Build history of the part. All positions in model axes, mm. Face numbers are marked on the shaded views. A direction names the side the tool comes from. Give positions to 0.01 mm unless a question says otherwise; leave off trailing zeros. Order: outer loops, then holes, each group sorted by start corner. A loop starts at its lowest first (then second) coordinate and runs counter-clockwise, first axis right, second up. Notation, with made-up numbers: M -18,88.25 L 40,88.25 A24 cw 40,104.25 Z; hole C -7.75,81 d5. An arc over 180 degrees is marked long. Use CSV: the item, a comma, the result in double quotes. Start each with the question number.
Item 1: Which spindle directions (+Z, -Z, +X, -X, +Y, -Y) get a long thin tool onto all of the face, cutting with end or side? Do the marked faces 1 and 2. Say none if no direction does.
Item 2: Pin check, flat tips, straight feed: P1, Ø4, axis at x = -5, y = -9.5, coming from the -Z side; P2, Ø1.4, axis at y = 0, z = 2.5, coming from the -X side; P3, Ø1, axis at y = 25, z = 2.5, coming from the +X side. Stop position of each tip, or through.
Item 3: Two-plate mould, pull along X, no slides. Class the marked faces 3, 4 and 5: pulls with the +X half, pulls with the -X half, needs draft (parallel to the pull), parting line crosses it, or undercut.
Item 4: Band-saw the part on C-C on x = -12. Write the cut outline in (y, z), plus the area to 3 significant figures.
Item 5: Band-saw the part on D-D on x = -2. Write the cut outline in (y, z).
Item 6: Band-saw the part on B-B on z = 2.5. Give the number of separate pieces and of enclosed holes in the cut face, plus the area to 3 significant figures.
Item 7: Wall check: line 1 along Y through (x, z) = (12.5, 0.7); line 2 along Y through (x, z) = (15.5, 2.5); line 3 along Z through (x, y) = (15, 25). Give the ranges that are in metal, low to high.
Item 8: Band-saw the part on A-A on y = -21.75. Write the cut outline in (x, z) (3 decimals).
from build123d import *

# Parameters (mm, degrees)
SKETCH1_W           = 33
SKETCH1_H           = 60
SKETCH1_R           = 4.58
SKETCH1_W_2         = 6
SKETCH1_H_2         = 6
BOSS_EXTRUDE1_DEPTH = 5
SKETCH2_R           = 0.85
CUT_EXTRUDE1_DEPTH  = 3
CUT_EXTRUDE2_START  = -3
SKETCH3_R           = 0.85
CUT_EXTRUDE2_DEPTH  = 3
FILLET1_R           = 3


with BuildPart() as part:
    # Sketch1 → Boss-Extrude1 (new body)
    with BuildSketch(Plane.XY):
        Rectangle(SKETCH1_W, SKETCH1_H)
        with Locations((-5.175, 21.75)):
            Circle(SKETCH1_R, mode=Mode.SUBTRACT)
        with Locations(Location((-5.175, -21.75, 0), (0, 0, 180))):
            Circle(SKETCH1_R, mode=Mode.SUBTRACT)
        with Locations((11.5, 0)):
            Rectangle(SKETCH1_W_2, SKETCH1_H_2, mode=Mode.SUBTRACT)
        with Locations((-11.5, 0)):
            Rectangle(SKETCH1_W_2, SKETCH1_H_2, mode=Mode.SUBTRACT)
    extrude(amount=BOSS_EXTRUDE1_DEPTH)

    # Sketch2 → Cut-Extrude1 (cut)
    with BuildSketch(Plane(origin=(16.5, 0, 0), x_dir=(0, 0, -1), z_dir=(1, 0, 0))):
        with Locations((-2.5, 0)):
            Circle(SKETCH2_R)
        with Locations((-2.5, -25)):
            Circle(SKETCH2_R)
        with Locations(Location((-2.5, 25, 0), (0, 0, 180))):
            Circle(SKETCH2_R)
    extrude(amount=-CUT_EXTRUDE1_DEPTH, mode=Mode.SUBTRACT)

    # Sketch3 → Cut-Extrude2 (cut)
    with BuildSketch(Plane.ZY.offset(16.5).offset(CUT_EXTRUDE2_START)):
        with Locations(Location((2.5, 0, 0), (0, 0, 180))):
            Circle(SKETCH3_R)
    extrude(amount=CUT_EXTRUDE2_DEPTH, mode=Mode.SUBTRACT)

    # Fillet1
    fillet1_edges = [part.edges().sort_by_distance(p)[0] for p in [
        (16.5, -30, 2.5),
        (-16.5, -30, 2.5),
        (-16.5, 30, 2.5),
        (16.5, 30, 2.5),
    ]]
    fillet(fillet1_edges, radius=FILLET1_R)


solid = part.part
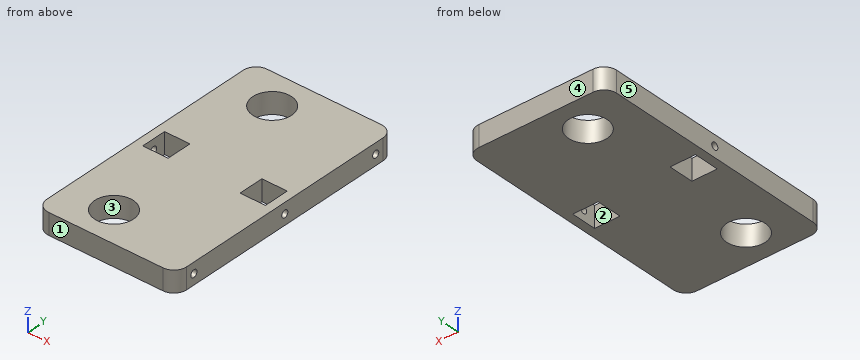
Model answer:
1,face 1,"+Z, -Z, +X, -X, -Y"
1,face 2,"+Z, -Z"
2,P1,"stops at z = 0"
2,P2,"stops at x = -8.5"
2,P3,"stops at x = 13.5"
3,face 3,"undercut"
3,face 4,"needs draft"
3,face 5,"pulls with the -X half"
4,outline,"M -30,0 L -3,0 L -3,5 L -30,5 Z; M 3,0 L 30,0 L 30,5 L 3,5 Z"
4,area,"270 mm^2"
5,outline,"M -30,0 L -25.05,0 L -25.05,5 L -30,5 Z; M -18.45,0 L 18.45,0 L 18.45,5 L -18.45,5 Z; M 25.05,0 L 30,0 L 30,5 L 25.05,5 Z"
6,separate pieces,"1"
6,enclosed holes,"2"
6,area,"1,750 mm^2"
7,line 1,"y = -30 to -3, 3 to 30"
7,line 2,"y = -29.24 to -25.85, -24.15 to -0.85, 0.85 to 24.15, 25.85 to 29.24"
7,line 3,"z = 0 to 1.65, 3.35 to 5"
8,outline,"M -16.5,0 L -9.755,0 L -9.755,5 L -16.5,5 Z; M -0.595,0 L 16.5,0 L 16.5,5 L -0.595,5 Z"
